Geometry check sheet. Reference: the model listing, model coordinates, mm. Round coordinates to 2 decimals unless told otherwise and drop trailing zeros. Loops run counter-clockwise (first coordinate to the right, second up) from the corner with the lowest first, then second, coordinate; pieces in that order, holes last. Notation, with made-up numbers: (-34, 27) - (-8, 27) arc R15 ccw to (-8, 36) - close; hole circle Ø3 at (13, 83.5). An arc over 180 degrees is marked (long way). Answer in a Markdown table with one row per item. Add a question column.
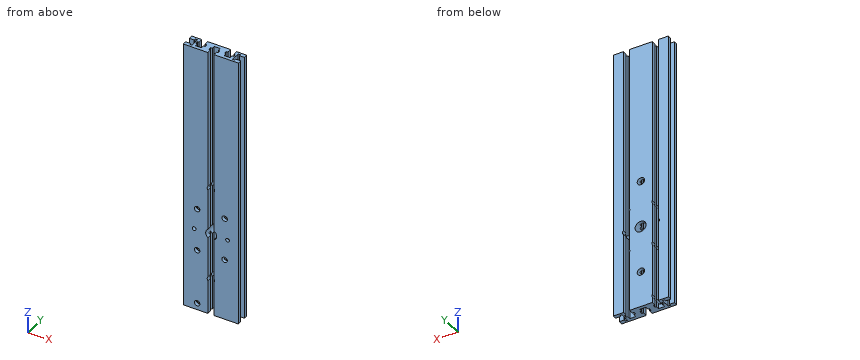
```python
from build123d import *

# Parameters (mm, degrees)
EXTRUDE_1_DEPTH         = 300
HOLE_WIZARD_12_0_12_1_D = 12
HOLE_WIZARD_8_0_8_1_D   = 8
HOLE_WIZARD_6_0_6_2_D   = 6
HOLE_WIZARD_M5_1_D      = 4.2


with BuildPart() as part:
    # 草图1 → 凸台-拉伸1 (new body)
    with BuildSketch(Plane.XY):
        Polygon((0, 0), (26.75, 0), (26.75, 4.796419132), (24.926505169, 4.796419132), (24.926505169, 8.023402897), (26.75, 8.023402897), (26.75, 11.5), (30, 11.5), (33.25, 11.5), (33.25, 8.023402897), (35.073494831, 8.023402897), (35.073494831, 4.796419132), (33.25, 4.796419132), (33.25, 0), (60, 0), (60, 4.25), (54.613325713, 4.25), (54.613325713, 2.4), (52.2, 2.4), (52.2, 12.6), (54.613325713, 12.6), (54.613325713, 10.75), (60, 10.75), (60, 15), (48.947608979, 15), (48.947608979, 10.003848618), (50.733802833, 10.003848618), (50.733802833, 7.094693738), (48.947608979, 7.094693738), (48.947608979, 3.5), (42.447608979, 3.5), (42.447608979, 7.094693738), (40.533802833, 7.094693738), (40.533802833, 10.003848618), (42.447608979, 10.003848618), (42.447608979, 15), (30, 15), (17.552391021, 15), (17.552391021, 10.003848618), (19.466197167, 10.003848618), (19.466197167, 7.094693738), (17.552391021, 7.094693738), (17.552391021, 3.5), (11.052391021, 3.5), (11.052391021, 7.094693738), (9.266197167, 7.094693738), (9.266197167, 10.003848618), (11.052391021, 10.003848618), (11.052391021, 15), (0, 15), (0, 10.75), (5.386674287, 10.75), (5.386674287, 12.6), (7.8, 12.6), (7.8, 2.4), (5.386674287, 2.4), (5.386674287, 4.25), (0, 4.25), align=None)
    extrude(amount=EXTRUDE_1_DEPTH)

    # Ø12.0 (12) 直径孔1 (through all)
    with Locations(Plane(origin=(0, 15, 0), x_dir=(1, 0, 0), z_dir=(0, 1, 0))):
        with Locations((30.31545922, -92)):
            Hole(HOLE_WIZARD_12_0_12_1_D / 2)

    # Ø8.0 (8) 直径孔1 (through all)
    with Locations(Plane(origin=(0, 15, 0), x_dir=(1, 0, 0), z_dir=(0, 1, 0))):
        with Locations((30, -40), (30, -144)):
            Hole(HOLE_WIZARD_8_0_8_1_D / 2)

    # Ø6.0 (6) 直径孔2 (through all)
    with Locations(Plane(origin=(0, 0, 0), x_dir=(-1, 0, 0), z_dir=(0, -1, 0))):
        with Locations((-15, -7.5), (-15, -68.3), (-15, -115.7), (-45, -68.3), (-45, -115.7)):
            Hole(HOLE_WIZARD_6_0_6_2_D / 2)

    # M5 螺纹孔的螺纹孔钻头1 (through all)
    with Locations(Plane(origin=(0, 0, 0), x_dir=(-1, 0, 0), z_dir=(0, -1, 0))):
        with Locations((-48.2, -92), (-11.8, -92)):
            Hole(HOLE_WIZARD_M5_1_D / 2)


solid = part.part
```
Q1. Cross-section at A-A, the plane x = 30. Enter the section's corners in (y, z).
Q2. Depth check by flat-ended pin: P1, Ø2.5, axis at y = 6, z = 245.5, coming from the +X side; P2, Ø1.1, axis at y = 5, z = 240, coming from the -X side. Enter the tip coordinate at first touch or a pass-through.
Q3. Scan lines: line 1 (X direction, y = 12.75, z = 40); line 2 (X direction, y = 3, z = 28); line 3 (X direction, y = 11, z = 199.5). Record each from-to range of solid material in increasing order. Write a range as from..to.
Check sheet entries:
| question | item | result |
|---|---|---|
| 1 | outline | (11.5, 0) - (15, 0) - (15, 36) - (11.5, 36) - close; (11.5, 44) - (15, 44) - (15, 86.01) - (11.5, 86.01) - close; (11.5, 97.99) - (15, 97.99) - (15, 140) - (11.5, 140) - close; (11.5, 148) - (15, 148) - (15, 300) - (11.5, 300) - close |
| 2 | P1 | x = 52.2 |
| 2 | P2 | x = 7.8 |
| 3 | line 1 | 0..11.05, 17.55..26, 34..42.45, 48.95..60 |
| 3 | line 2 | 0..5.39, 7.8..26.75, 33.25..52.2, 54.61..60 |
| 3 | line 3 | 0..5.39, 7.8..11.05, 17.55..26.75, 33.25..42.45, 48.95..52.2, 54.61..60 |
